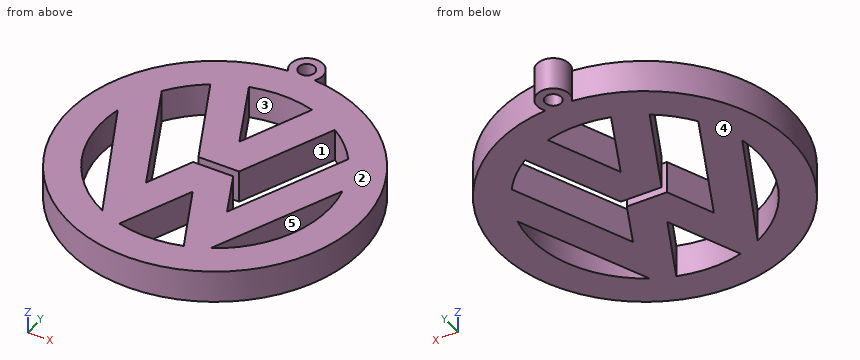
```python
from build123d import *

# Parameters (mm, degrees)
F0_R     = 1.241195
F1_DEPTH = 5


with BuildPart() as f1:
    # F0 (on Top) → F1 (new body)
    with BuildSketch(Plane.XY):
        with BuildLine():
            ThreePointArc((2.028342, 22.408387), (0, 26.323733), (-2.028342, 22.408387))
            ThreePointArc((-2.028342, 22.408387), (0, -22.5), (2.028342, 22.408387))
        make_face()
        with BuildLine():
            ThreePointArc((-7.988275, -15.570403), (-15.882311, -7.348618), (-17.038951, 3.990506))
            Line((-17.038951, 3.990506), (-7.988275, -15.570403))
        make_face(mode=Mode.SUBTRACT)
        with BuildLine():
            ThreePointArc((5.022585, -16.76376), (0.186737, -17.499004), (-4.6637, -16.867125))
            Line((-4.6637, -16.867125), (0.201713, -6.156514))
            Line((0.201713, -6.156514), (5.022585, -16.76376))
        make_face(mode=Mode.SUBTRACT)
        with BuildLine():
            Line((8.288617, -15.412619), (17.083899, 3.793469))
            ThreePointArc((17.083899, 3.793469), (15.91099, -7.286317), (8.288617, -15.412619))
        make_face(mode=Mode.SUBTRACT)
        with BuildLine():
            Line((3.280106, 0.620191), (9.634679, 14.609003))
            ThreePointArc((9.634679, 14.609003), (12.181654, 12.564128), (14.304266, 10.081566))
            Line((14.304266, 10.081566), (6.233971, -7.599009))
            Line((6.233971, -7.599009), (3.134064, -0.652507))
            Line((3.134064, -0.652507), (-2.938647, -0.652507))
            Line((-2.938647, -0.652507), (-6.040588, -7.544222))
            Line((-6.040588, -7.544222), (-14.098893, 10.366833))
            ThreePointArc((-14.098893, 10.366833), (-11.921222, 12.811498), (-9.326312, 14.807765))
            Line((-9.326312, 14.807765), (-2.878222, 0.620191))
            Line((-2.878222, 0.620191), (3.280106, 0.620191))
        make_face(mode=Mode.SUBTRACT)
        with BuildLine():
            ThreePointArc((-4.6819, 16.862082), (0.121059, 17.499581), (4.914738, 16.795694))
            Line((4.914738, 16.795694), (0.110725, 6.122414))
            Line((0.110725, 6.122414), (-4.6819, 16.862082))
        make_face(mode=Mode.SUBTRACT)
        with Locations((0, 23.84067)):
            Circle(F0_R, mode=Mode.SUBTRACT)
    extrude(amount=F1_DEPTH)


solid = f1.part
```
Work out the finished part from the listing and answer in its coordinate system (mm). Face numbers are marked on the shaded views. A direction names the side the tool comes from. Give positions to 0.01 mm unless a question says otherwise; leave off trailing zeros. Write each loop counter-clockwise with the first axis right and the second up, starting at its lowest first coordinate (ties: lowest second). Pieces come first, ordered by that corner, then holes. Notation, with made-up numbers: (31.5, 67.5) - (54.5, 67.5) arc R17 ccw to (54.5, 72.5) - close; hole circle Ø4 at (-7, 55.25). An arc over 180 degrees is marked (long way). Use one line per item in the form item = value.
1. A cutting plane is placed at C-C (y = -9). Write down the section's boundary in (x, z), and give its area (3 significant figures).
Filled in:
outline = (-20.62, 0) - (-15.01, 0) - (-15.01, 5) - (-20.62, 5) - close; (-11.03, 0) - (-1.09, 0) - (-1.09, 5) - (-11.03, 5) - close; (1.49, 0) - (11.23, 0) - (11.23, 5) - (1.49, 5) - close; (15.01, 0) - (20.62, 0) - (20.62, 5) - (15.01, 5) - close
area = 154 mm^2
2. A cutting plane is placed at B-B (z = 2.7). Write down the section's boundary in (x, y).
Filled in:
outline = (-2.03, 22.41) arc R22.5 ccw (long way) to (2.03, 22.41) arc R2.48 ccw (long way) to start; hole (-17.04, 3.99) arc R17.5 ccw to (-7.99, -15.57) - close; hole (-14.1, 10.37) - (-6.04, -7.54) - (-2.94, -0.65) - (3.13, -0.65) - (6.23, -7.6) - (14.3, 10.08) arc R17.5 ccw to (9.63, 14.61) - (3.28, 0.62) - (-2.88, 0.62) - (-9.33, 14.81) arc R17.5 ccw to start; hole (-4.68, 16.86) - (0.11, 6.12) - (4.91, 16.8) arc R17.5 ccw to start; hole (-4.66, -16.87) arc R17.5 ccw to (5.02, -16.76) - (0.2, -6.16) - close; hole circle Ø2.48 at (0, 23.84); hole (8.29, -15.41) arc R17.5 ccw to (17.08, 3.79) - close
3. A cutting plane is placed at A-A (y = -3). Write down the section's boundary in (x, z), and give its area (3 significant figures).
Filled in:
outline = (-22.3, 0) - (-17.24, 0) - (-17.24, 5) - (-22.3, 5) - close; (-13.8, 0) - (-8.09, 0) - (-8.09, 5) - (-13.8, 5) - close; (-4, 0) - (4.18, 0) - (4.18, 5) - (-4, 5) - close; (8.33, 0) - (13.97, 0) - (13.97, 5) - (8.33, 5) - close; (17.24, 0) - (22.3, 0) - (22.3, 5) - (17.24, 5) - close
area = 148 mm^2
4. Determine the mould class of the marked faces 3, 4 and 5 for opening direction Y: released by +Y, released by -Y, zero draft, split by the parting line, or undercut.
Filled in:
face_3 = undercut
face_4 = zero draft
face_5 = undercut
5. For the marked faces 1 and 2, determine the directions among +Z, -Z, +X, -X, +Y, -Y from which every point of the face is accessible in a straight line to the end or side of a thin tool.
Filled in:
face_1 = +Z, -Z
face_2 = +Z, +X, -X, +Y, -Y
6. Each of these flat-tipped pins is pushed along its axis until it touches: pin 1 Ø2 at (x, z) = (1.5, 1.5) entering from -Y; pin 2 Ø2.5 at (x, z) = (1.5, 3.5) entering from +Y; pin 3 Ø3 at (x, z) = (-16.5, 1.5) entering from +Y. Where does it stop, or does it pass through?
Filled in:
pin_1 = -22.49
pin_2 = 26.31
pin_3 = 16.77
7. A cutting plane is placed at D-D (y = 9.5). Write down the section's boundary in (x, z).
Filled in:
outline = (-20.4, 0) - (-13.71, 0) - (-13.71, 5) - (-20.4, 5) - close; (-6.91, 0) - (-1.4, 0) - (-1.4, 5) - (-6.91, 5) - close; (1.63, 0) - (7.31, 0) - (7.31, 5) - (1.63, 5) - close; (14.04, 0) - (20.4, 0) - (20.4, 5) - (14.04, 5) - close
8. Consider L1, parallel to X at y = -13.5, z = 2.8; L2, parallel to X at y = -10, z = 0.4; L3, parallel to Y at x = 4, z = 4.8. Determine where each line is inside the solid, lowest interval first.
Filled in:
L1 = -18 to -11.14, -8.95 to -3.13, 3.54 to 9.16, 11.14 to 18
L2 = -20.16 to -14.36, -10.57 to -1.54, 1.95 to 10.77, 14.36 to 20.16
L3 = -22.14 to -17.04, -14.51 to -2.59, 2.2 to 14.76, 17.04 to 22.14
